Input: part model. Units: mm. Frame: model coordinates. A direction names the side the tool comes from. Give positions to 0.01 mm unless a question says otherwise; leave off trailing zeros. Loops run counter-clockwise (first coordinate to the right, second up) from the corner with the lowest first, then second, coordinate; pieces in that order, holes last. Notation, with made-up numbers: (-17.5, 23.5) - (2.5, 23.5) arc R20 ccw to (2.5, 59.5) - close; hole circle Ø3 at (58, 4.25). An arc over 180 degrees is marked (long way). Answer as a JSON object with one key per item and string values. Group by question number.
(1) Material intervals for L1, parallel to X at y = -5, z = 7.75; L2, parallel to Z at x = -8.75, y = -9.2; L3, parallel to Y at x = -1.5, z = 9.5, sorted ascending.
(2) Section query D-D (y = -9.75). Count the separate pieces of the cut face and the enclosed holes in it, plus the area to 3 significant figures.
(3) Pin query (flat end, axial travel): P1, Ø1.8, axis at x = 9.5, z = 4, coming from the +Y side; P2, Ø2.5, axis at x = 8.75, z = 4, coming from the +Y side; P3, Ø1.5, axis at y = -2, z = 10, coming from the +X side; P4, Ø1.8, axis at x = -8.75, z = 4, coming from the -Y side. Return the tip coordinate at first contact, or that it passes through.
(4) Mould query, pull axis X, two halves, no side actions, for faces 1 (the cylindrical face through (-7.551, -7.715, 3.945)), 2 (the flat face through (-1, -1, 0)), 3 (the cylindrical face through (-8.62, -9.45, 4.99)). Classes: +X half, -X half, draft (parallel to the pull), parting line (faces both ways), or undercut.
(5) Section query A-A (y = -3.75). Return loops of the section in (x, z).
(6) Section query B-B (z = 3.5). Return loops of the section in (x, y).
(7) Section query C-C (x = 8.75). Return loops of the section in (y, z), plus the area to 3 significant figures.
(8) Access query for faces 4 (the flat face through (-10, -8, 4)), 5 (the flat face through (10, -8, 4)), 6 (the flat face through (5.75, -7, 6)). Directions: +Z, -Z, +X, -X, +Y, -Y. A direction counts if a zero-diameter tool reaches every point of the face in a straight line with its end or side. Return the directions, or none.
```python
from build123d import *

# Parameters (mm, degrees)
SALIENTE_EXTRUIR1_DEPTH    = 11.5
REDONDEO1_R                = 0.5
CORTAR_EXTRUIR1_DEPTH      = 19.284214503
CORTAR_EXTRUIR2_DEPTH      = 19.284214567
CORTAR_EXTRUIR2_DEPTH_BACK = 19.284214567
CROQUIS4_R                 = 1


with BuildPart() as part:
    # Croquis1 → Saliente-Extruir1 (new body)
    with BuildSketch(Plane.XY):
        with BuildLine():
            Line((7.25, 0), (0, 0))
            Line((0, 0), (0, -1.5))
            Line((0, -1.5), (4.25, -1.5))
            ThreePointArc((4.25, -1.5), (5.310660172, -1.939339828), (5.75, -3))
            Line((5.75, -3), (5.75, -11))
            Line((5.75, -11), (11.75, -11))
            Line((11.75, -11), (11.75, -8))
            Line((11.75, -8), (8.25, -8))
            ThreePointArc((8.25, -8), (7.542893219, -7.707106781), (7.25, -7))
            Line((7.25, -7), (7.25, 0))
        make_face()
    saliente_extruir1 = extrude(amount=SALIENTE_EXTRUIR1_DEPTH)

    # Simetría1: Saliente-Extruir1 across plane
    add(saliente_extruir1.mirror(Plane(origin=(0, 0, 11.5), x_dir=(0, 0, 1), z_dir=(1, 0, 0))))

    # Redondeo1
    redondeo1_edges = [part.edges().sort_by_distance(p)[0] for p in [
        (7.25, 0, 5.75),
        (-7.25, 0, 5.75),
    ]]
    fillet(redondeo1_edges, radius=REDONDEO1_R)

    # Croquis3 → Cortar-Extruir1 (cut, symmetric)
    with BuildSketch(Plane(origin=(0, -8, 0), x_dir=(1, 0, 0), z_dir=(0, 1, 0))):
        with BuildLine():
            Line((8.25, -11.5), (8.25, -7.968626967))
            ThreePointArc((8.25, -7.968626967), (7.75, -8), (7.25, -7.968626967))
            Line((7.25, -7.968626967), (7.25, -11.5))
            Line((7.25, -11.5), (8.25, -11.5))
        make_face()
        with BuildLine():
            Line((11.75, -11.5), (11.75, -4))
            ThreePointArc((11.75, -4), (10.75, -6.645751311), (8.25, -7.968626967))
            Line((8.25, -7.968626967), (8.25, -11.5))
            Line((8.25, -11.5), (11.75, -11.5))
        make_face()
        with BuildLine():
            Line((11.75, 0), (8.25, 0))
            Line((8.25, 0), (8.25, -0.031373033))
            ThreePointArc((8.25, -0.031373033), (10.75, -1.354248689), (11.75, -4))
            Line((11.75, -4), (11.75, 0))
        make_face()
    cortar_extruir1 = extrude(amount=CORTAR_EXTRUIR1_DEPTH, both=True, mode=Mode.SUBTRACT)

    # Simetría2: Cortar-Extruir1 across plane
    add(cortar_extruir1.mirror(Plane(origin=(0, 0, 0), x_dir=(0, 0, 1), z_dir=(1, 0, 0))), mode=Mode.SUBTRACT)

    # Croquis4 → Cortar-Extruir2 (cut, two sides: drawn at the far end of the back side and taken through both)
    with BuildSketch(Plane(origin=(0, -8, 0), x_dir=(1, 0, 0), z_dir=(0, 1, 0)).offset(-CORTAR_EXTRUIR2_DEPTH_BACK)):
        with Locations(Location((8.75, -4, 0), (0, 0, 180))):
            Circle(CROQUIS4_R)
        with Locations(Location((-8.75, -4, 0), (0, 0, 60))):
            Circle(CROQUIS4_R)
    extrude(amount=CORTAR_EXTRUIR2_DEPTH + CORTAR_EXTRUIR2_DEPTH_BACK, mode=Mode.SUBTRACT)


solid = part.part
```
Recorded:
{
 "1": {"L1": "x = -7.25 to -5.75, 5.75 to 7.25", "L2": "z = 0.13 to 3, 5 to 7.87", "L3": "y = -1.5 to 0"},
 "2": {"separate pieces": "2", "enclosed holes": "2", "area": "86.5 mm^2"},
 "3": {"P1": "stops at y = -8", "P2": "stops at y = -7.66", "P3": "stops at x = 7.25", "P4": "passes through"},
 "4": {"face 1": "-X half", "face 2": "draft", "face 3": "undercut"},
 "5": {"outline": "(-7.25, 0) - (-5.75, 0) - (-5.75, 11.5) - (-7.25, 11.5) - close; (5.75, 0) - (7.25, 0) - (7.25, 11.5) - (5.75, 11.5) - close"},
 "6": {"outline": "(-11.72, -11) - (-9.62, -11) - (-9.62, -8) - (-11.72, -8) - close; (-7.88, -11) - (-5.75, -11) - (-5.75, -3) arc R1.5 cw to (-4.25, -1.5) - (4.25, -1.5) arc R1.5 cw to (5.75, -3) - (5.75, -11) - (7.88, -11) - (7.88, -7.93) arc R1 cw to (7.25, -7) - (7.25, -0.5) arc R0.5 ccw to (6.75, 0) - (-6.75, 0) arc R0.5 ccw to (-7.25, -0.5) - (-7.25, -7) arc R1 cw to (-7.88, -7.93) - close; (9.62, -11) - (11.72, -11) - (11.72, -8) - (9.62, -8) - close"},
 "7": {"outline": "(-11, 0.13) - (-8, 0.13) - (-8, 3) - (-11, 3) - close; (-11, 5) - (-8, 5) - (-8, 7.87) - (-11, 7.87) - close", "area": "17.2 mm^2"},
 "8": {"face 4": "+Z, -Z, -X, +Y", "face 5": "+Z, -Z, +X, +Y", "face 6": "+Z, -Z, -Y"}
}
